Input: part model. Units: mm. Frame: model coordinates. A direction names the side the tool comes from. Round coordinates to 2 decimals unless told otherwise and drop trailing zeros. Write each loop counter-clockwise with the first axis right and the second up, starting at its lowest first coordinate (ties: lowest second). Pieces come first, ordered by that corner, then holes. Notation, with made-up numbers: M -32.75,6 L 18.25,6 A33 ccw 18.25,34 Z; hole C 45.5,71.5 d3. An arc over 180 degrees is marked long. Write each question's results on one line, items separated by ' | '. Start each with the question number.
Autodesk Inventor part; units mm, degrees
ref_plane "YZ Plane" through (0, 0, 0) normal (1, 0, 0) x (0, 1, 0)
ref_plane "XZ Plane" through (0, 0, 0) normal (0, 1, 0) x (-1, 0, 0)
ref_plane "XY Plane" through (0, 0, 0) normal (0, 0, 1) x (1, 0, 0)
sketch "Boceto1" plane through (0, 0, 0) normal (0, 0, 1) x (1, 0, 0)
  line L0 (0, 0) -> (8, 0)
  line L1 (8, 0) -> (8, 8)
  line L2 (8, 8) -> (0, 8)
  line L3 (0, 8) -> (0, 0)
  line L4 (8, 0) -> (32, 0)
  line L5 (32, 0) -> (32, 4)
  line L6 (32, 4) -> (8, 4)
  line L7 (8, 4) -> (8, 0)
  dimension "d0" = 8
  dimension "d2" = 24
  dimension "d3" = 4
  dimension "d23" = 8
extrude "Extrusión1" add sketch "Boceto1" along normal blind 1.9
fillet "Empalme5" radius 4 3 edges at (0, 0, 0.95) (0, 8, 0.95) (8, 8, 0.95)
fillet "Empalme6" radius 2 2 edges at (32, 4, 0.95) (32, 0, 0.95)
sketch "Boceto2" plane through (0, 0, 1.9) normal (0, 0, 1) x (1, 0, 0)
  arc A0 (8, 4) -> (4, 0) centre (4, 4) ccw
  point P0 (0, 0)
hole "Hole1" at (4, 4, 1.9) direction (0, 0, -1) diameter 1 end through all
sketch "Boceto3" plane through (0, 0, 1.9) normal (0, 0, 1) x (1, 0, 0)
  circle A0 centre (4, 4) radius 0.5
  line L0 (8, 4) -> (30, 4)
  arc A1 (8, 4) -> (4, 0) centre (4, 4) ccw
  line L1 (30, 0) -> (4, 0)
  line L2 (22.5, 4) -> (22.5, 0)
  point P0 (0, 0)
  dimension "d19" = 14.5
extrude "Extrusión2" add sketch "Boceto3" along normal blind 2
fillet "Empalme7" radius 2 2 edges at (22.5, 0, 2.9) (22.5, 4, 2.9)
properties part number "Traba"
1. Contact query for flat-ended pins moving along their axis: P1, Ø1, axis at y = 6, z = 3.5, coming from the +X side; P2, Ø1.5, axis at x = 4.5, y = 4, coming from the -Z side. Output: stop coordinate, or through.
2. Draft query along X for faces 1 (the face through (4.464, 3.814, 1.923)), 2 (the face through (1.141, 1.203, 0.963)), 3 (the face through (21.9, 0.57, 2.91)). Return one class per face: +X half, -X half, draft (parallel to the pull), parting line (faces both ways), or undercut.
3. Access query for faces 4 (the face through (31.4, 0.57, 0.96)), 5 (the face through (16, 4, 1)), 6 (the face through (21.93, 3.4, 2.91)). Directions: +Z, -Z, +X, -X, +Y, -Y. A direction counts if a zero-diameter tool reaches every point of the face in a straight line with its end or side. Return the directions, or none.
4. Line query: L1, parallel to Y at x = 4, z = 2.4; L2, parallel to Y at x = 15, z = 3.4; L3, parallel to Z at x = 29.5, y = 1.5. Output: solid intervals per line, ascending. Write a range as from..to.
5. Cut plane C-C on x = 20. Output: boundary loops of the cut face in (y, z), and give its area (3 significant figures).
Answers follow:
1) P1: stops at x = 7.71 | P2: stops at z = 0
2) face 1: undercut | face 2: -X half | face 3: +X half
3) face 4: +Z, -Z, +X, -Y | face 5: +Z, -Z, +X, +Y | face 6: +Z, +X, +Y
4) L1: y = 0..3.5, 4.5..8 | L2: y = 0..4 | L3: z = 0..1.9
5) outline: M 0,0 L 4,0 L 4,3.9 L 0,3.9 Z | area: 15.6 mm2
